For this review, take the finished solid that the model builds, in its own axes (mm). Give positions to 0.01 mm unless a question says otherwise; leave off trailing zeros. Write each loop counter-clockwise with the first axis right and the second up, starting at its lowest first coordinate (ties: lowest second). Pieces come first, ordered by that corner, then holes.
from build123d import *

# Parameters (mm, degrees)
SKETCH1_W           = 1092.2
SKETCH1_H           = 762
BOSS_EXTRUDE1_DEPTH = 25.4
CUT_EXTRUDE1_DEPTH  = 667.356788815
SWEEP1_PROFILE_R    = 6.35


with BuildPart() as part:
    # Sketch1 → Boss-Extrude1 (new body)
    with BuildSketch(Plane(origin=(0, 0, 0), x_dir=(1, 0, 0), z_dir=(0, 1, 0))):
        Rectangle(SKETCH1_W, SKETCH1_H)
    extrude(amount=BOSS_EXTRUDE1_DEPTH)

    # Sketch2 → Cut-Extrude1 (cut, through all)
    with BuildSketch(Plane(origin=(0, 25.4, 0), x_dir=(1, 0, 0), z_dir=(0, 1, 0))):
        Polygon((-546.1, 183.043938976), (-546.1, 132.243938976), (-546.1, 81.443938976), (-533.4, 81.443938976), (-533.4, 183.043938976), align=None)
        Polygon((-546.1, -122.927339743), (-546.1, -173.727339743), (-533.4, -173.727339743), (-533.4, -72.127339743), (-546.1, -72.127339743), align=None)
    extrude(amount=-CUT_EXTRUDE1_DEPTH, mode=Mode.SUBTRACT)

    # Sweep1: sweep along a path in Sketch3
    with BuildLine(Plane(origin=(508, 0, 0), x_dir=(0, 0, -1), z_dir=(1, 0, 0))) as sweep1_path:
        Line((-330.2, 25.4), (-330.2, 50.8))
        Line((-330.2, 50.8), (330.2, 50.8))
        Line((330.2, 50.8), (330.2, 25.4))
    # Sweep1 profile (on start of the path) → Sweep1 (sweep)
    with BuildSketch(Plane(origin=(508, 25.4, 330.2), x_dir=(0, 0, 1), z_dir=(0, 1, 0))):
        Circle(SWEEP1_PROFILE_R)
    sweep(path=sweep1_path.line, transition=Transition.RIGHT)


solid = part.part
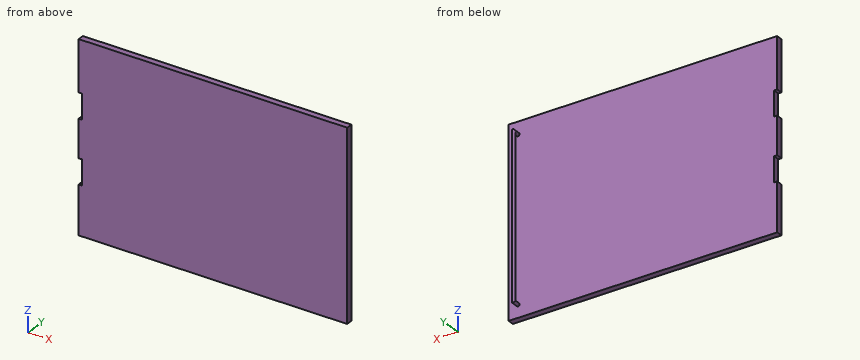
(1) Clearance check with flat-ended pins moving along their axes: pin 1 Ø10 at (y, z) = (38.5, -63) entering from +X; pin 2 Ø20.5 at (y, z) = (12, 134) entering from -X; pin 3 Ø1 at (x, z) = (134.5, -36.5) entering from +Y; pin 4 Ø3 at (y, z) = (48.5, 210.5) entering from +X. State where each tip first meets the part, or that it passes through.
(2) We need section C-C (z = 147.5). Write out the cut boundary in (x, y).
(3) We need section B-B (x = -43). Write out the cut boundary in (y, z), and give its area (3 significant figures).
(4) For L1, parallel to Y at x = 14.5, z = 250; L2, parallel to X at y = 11.5, z = -103; L3, parallel to X at y = 53, z = -221, list the stretches that pass through material, from the lowest coordinate up.
(5) We need section A-A (z = 250.5). Write out the cut boundary in (x, y), and give its area (3 significant figures).
The answers:
1. pin 1: passes through
1. pin 2: stops at x = -533.4
1. pin 3: stops at y = 25.4
1. pin 4: stops at x = 514.3
2. outline: (-533.4, 0) - (546.1, 0) - (546.1, 25.4) - (-533.4, 25.4) - close; circle Ø12.7 at (508, 50.8)
3. outline: (0, -381) - (25.4, -381) - (25.4, 381) - (0, 381) - close
3. area: 19,400 mm2
4. L1: y = 0 to 25.4
4. L2: x = -533.4 to 546.1
4. L3: x = 502.04 to 513.96
5. outline: (-546.1, 0) - (546.1, 0) - (546.1, 25.4) - (-546.1, 25.4) - close; circle Ø12.7 at (508, 50.8)
5. area: 27,900 mm2
